from build123d import *
from OCP.BRepFilletAPI import BRepFilletAPI_MakeChamfer

# Parameters (mm, degrees)
CROQUIS2_W              = 10
CROQUIS2_H              = 20
SALIENTE_EXTRUIR1_DEPTH = 0.7
CROQUIS3_W              = 7
CROQUIS3_H              = 17
CORTAR_EXTRUIR1_DEPTH   = 0.6
CROQUIS4_W              = 5
CROQUIS4_H              = 14
SALIENTE_EXTRUIR2_DEPTH = 0.6
CHAFL_N1_SIZE           = 0.2
CHAFL_N1_SIZE2          = 0.368354177
CROQUIS5_R              = 0.5
SALIENTE_EXTRUIR3_DEPTH = 0.4
CHAFL_N2_SIZE           = 0.2
CHAFL_N2_SIZE2          = 0.25143446


with BuildPart() as part:
    # Croquis2 → Saliente-Extruir1 (new body)
    with BuildSketch(Plane.XY):
        Rectangle(CROQUIS2_W, CROQUIS2_H)
    extrude(amount=SALIENTE_EXTRUIR1_DEPTH)

    # Croquis3 → Cortar-Extruir1 (cut)
    with BuildSketch(Plane.XY.offset(0.7)):
        Rectangle(CROQUIS3_W, CROQUIS3_H)
    extrude(amount=-CORTAR_EXTRUIR1_DEPTH, mode=Mode.SUBTRACT)

    # Croquis4 → Saliente-Extruir2 (add)
    with BuildSketch(Plane.XY.offset(0.1)):
        Rectangle(CROQUIS4_W, CROQUIS4_H)
    extrude(amount=SALIENTE_EXTRUIR2_DEPTH)

    # Chaflán1: one chamfer whose edges measure the first distance from different faces: ONE call of the kernel's chamfer builder (chamfer() names one face for all edges)
    chafl_n1_edges_1 = [part.edges().sort_by_distance(p)[0] for p in [
        (2.5, 0, 0.7),
    ]]
    chafl_n1_side_1 = [part.faces().sort_by_distance(p)[0] for p in [
        (2.5, 0, 0.4),
    ]]
    chafl_n1_edges_2 = [part.edges().sort_by_distance(p)[0] for p in [
        (0, 7, 0.7),
    ]]
    chafl_n1_side_2 = [part.faces().sort_by_distance(p)[0] for p in [
        (0, 7, 0.4),
    ]]
    chafl_n1_edges_3 = [part.edges().sort_by_distance(p)[0] for p in [
        (-2.5, 0, 0.7),
    ]]
    chafl_n1_side_3 = [part.faces().sort_by_distance(p)[0] for p in [
        (-2.5, 0, 0.4),
    ]]
    chafl_n1_edges_4 = [part.edges().sort_by_distance(p)[0] for p in [
        (0, -7, 0.7),
    ]]
    chafl_n1_side_4 = [part.faces().sort_by_distance(p)[0] for p in [
        (0, -7, 0.4),
    ]]
    chafl_n1 = BRepFilletAPI_MakeChamfer(part.part.solid().wrapped)
    for e in chafl_n1_edges_1:
        chafl_n1.Add(CHAFL_N1_SIZE, CHAFL_N1_SIZE2, e.wrapped, chafl_n1_side_1[0].wrapped)  # the first distance lies on this face
    for e in chafl_n1_edges_2:
        chafl_n1.Add(CHAFL_N1_SIZE, CHAFL_N1_SIZE2, e.wrapped, chafl_n1_side_2[0].wrapped)  # the first distance lies on this face
    for e in chafl_n1_edges_3:
        chafl_n1.Add(CHAFL_N1_SIZE, CHAFL_N1_SIZE2, e.wrapped, chafl_n1_side_3[0].wrapped)  # the first distance lies on this face
    for e in chafl_n1_edges_4:
        chafl_n1.Add(CHAFL_N1_SIZE, CHAFL_N1_SIZE2, e.wrapped, chafl_n1_side_4[0].wrapped)  # the first distance lies on this face
    add(Compound.cast(chafl_n1.Shape()), mode=Mode.REPLACE)

    # Croquis5 → Saliente-Extruir3 (add)
    with BuildSketch(Plane.XY.offset(0.7)):
        with Locations(Location((-4.208071118, 0, 0), (0, 0, 180))):
            Circle(CROQUIS5_R)
    extrude(amount=SALIENTE_EXTRUIR3_DEPTH)

    # Chaflán2
    chafl_n2_edges = [part.edges().sort_by_distance(p)[0] for p in [
        (-3.708071118, 0, 1.1),
    ]]
    chafl_n2_side = [part.faces().sort_by_distance(p)[0] for p in [
        (-3.708071118, 0, 0.9),
    ]]
    chamfer(chafl_n2_edges, length=CHAFL_N2_SIZE, length2=CHAFL_N2_SIZE2, reference=chafl_n2_side[0])


solid = part.part
The listing builds one solid part. Answer for the finished solid, in the listing's coordinates (mm). Coordinates: 2 decimals unless noted, no trailing zeros. Write each loop counter-clockwise with the first axis right and the second up, starting at its lowest first coordinate (ties: lowest second). Pieces come first, ordered by that corner, then holes. Notation, with made-up numbers: (85, 5.25) -> (103, 5.25) arc R20 ccw to (103, 39.25) -> close; hole circle Ø7 at (63, 81.5). An arc over 180 degrees is marked (long way). One line per question, with ' | ' between items.
1. Given pin 1 Ø1 at (x, y) = (1, 4) entering from -Z; pin 2 Ø2 at (x, y) = (-0.5, -2.5) entering from +Z, each flat-ended and moving along its own axis, determine where each tip first touches the part or whether it passes through.
Verdict:
pin 1: stops at z = 0 | pin 2: stops at z = 0.7
2. Section A-A (y = 0) is taken. Determine the outline of the cut face in (x, z), and give its area (3 significant figures).
Verdict:
outline: (-5, 0) -> (5, 0) -> (5, 0.7) -> (3.5, 0.7) -> (3.5, 0.1) -> (2.5, 0.1) -> (2.5, 0.5) -> (2.13, 0.7) -> (-2.13, 0.7) -> (-2.5, 0.5) -> (-2.5, 0.1) -> (-3.5, 0.1) -> (-3.5, 0.7) -> (-3.71, 0.7) -> (-3.71, 0.9) -> (-3.96, 1.1) -> (-4.46, 1.1) -> (-4.71, 0.9) -> (-4.71, 0.7) -> (-5, 0.7) -> close | area: 6.08 mm^2
3. Straight lines are drawn through the part: line 1 (X direction, y = -1, z = 0.3); line 2 (Y direction, x = 0.5, z = 0.15); line 3 (Y direction, x = -2.75, z = 0.5). For each, find the intervals that lie inside material, in ascending order.
Verdict:
line 1: x = -5 to -3.5, -2.5 to 2.5, 3.5 to 5 | line 2: y = -10 to -8.5, -7 to 7, 8.5 to 10 | line 3: y = -10 to -8.5, 8.5 to 10
4. Section D-D (x = 3.75) is taken. Determine the outline of the cut face in (y, z).
Verdict:
outline: (-10, 0) -> (10, 0) -> (10, 0.7) -> (-10, 0.7) -> close
5. Section C-C (y = 4.25) is taken. Determine the outline of the cut face in (x, z), and give its area (3 significant figures).
Verdict:
outline: (-5, 0) -> (5, 0) -> (5, 0.7) -> (3.5, 0.7) -> (3.5, 0.1) -> (2.5, 0.1) -> (2.5, 0.5) -> (2.13, 0.7) -> (-2.13, 0.7) -> (-2.5, 0.5) -> (-2.5, 0.1) -> (-3.5, 0.1) -> (-3.5, 0.7) -> (-5, 0.7) -> close | area: 5.73 mm^2
6. Section B-B (x = 1.5) is taken. Determine the outline of the cut face in (y, z).
Verdict:
outline: (-10, 0) -> (10, 0) -> (10, 0.7) -> (8.5, 0.7) -> (8.5, 0.1) -> (7, 0.1) -> (7, 0.5) -> (6.63, 0.7) -> (-6.63, 0.7) -> (-7, 0.5) -> (-7, 0.1) -> (-8.5, 0.1) -> (-8.5, 0.7) -> (-10, 0.7) -> close
